For this review, use the dimensioned drawing (mm, ordinates from the lowest corner) and the shaded views. A direction names the side the tool comes from. Coordinates: 2 decimals unless noted, no trailing zeros. Loops run counter-clockwise (first coordinate to the right, second up) from the corner with the lowest first, then second, coordinate; pieces in that order, holes last. Notation, with made-up numbers: (88.5, 77) - (129.5, 77) arc R20 ccw to (129.5, 106) - close; hole circle Ø5 at (28.25, -16.75). An arc over 180 degrees is marked (long way). Use a Markdown table: item, result. Add a question column.
1) To check wall thickness, follow L1, parallel to Y at x = 19.05, z = 35.5; L2, parallel to X at y = 19, z = 30; L3, parallel to Z at x = 30.5, y = 83.5. State the ranges of each line that lie inside material, in increasing order. Write a range as [from, to].
2) Add section A-A, the plane z = 7.5. Give the boundary of the cut face in (x, y), and give its area (3 significant figures).
3) The part is to be moulded in two halves that separate along Y. For the marked faces 1, 2, 3 and 4, say which applies: pulls with the +Y half, pulls with the -Y half, needs draft (parallel to the pull), parting line crosses it, or undercut.
4) Add section C-C, the plane x = 19.05. Give the boundary of the cut face in (y, z) (3 decimals).
5) Clearance check with flat-ended pins moving along their axes: pin 1 (11.5 mm diameter, centred on x = 133.35, y = 19.05, fed in from -Z); pin 2 (14.5 mm diameter, centred on x = 91, y = 90.5, fed in from +Z); pin 3 (10 mm diameter, centred on x = 63, y = 74.5, fed in from -Z). State where each tip first meets the part, or that it passes through.
6) Add section B-B, the plane y = 19.05. Give the boundary of the cut face in (x, z).
7) For the marked faces 5, 6 and 7, list the 3-axis set-ups (+Z, -Z, +X, -X, +Y, -Y) from which the entire face can be reached by the end or side of a thin tool; tool diameter is ignored.
8) Add section D-D, the plane y = 42.5. Give the boundary of the cut face in (x, z), and give its area (3 significant figures).
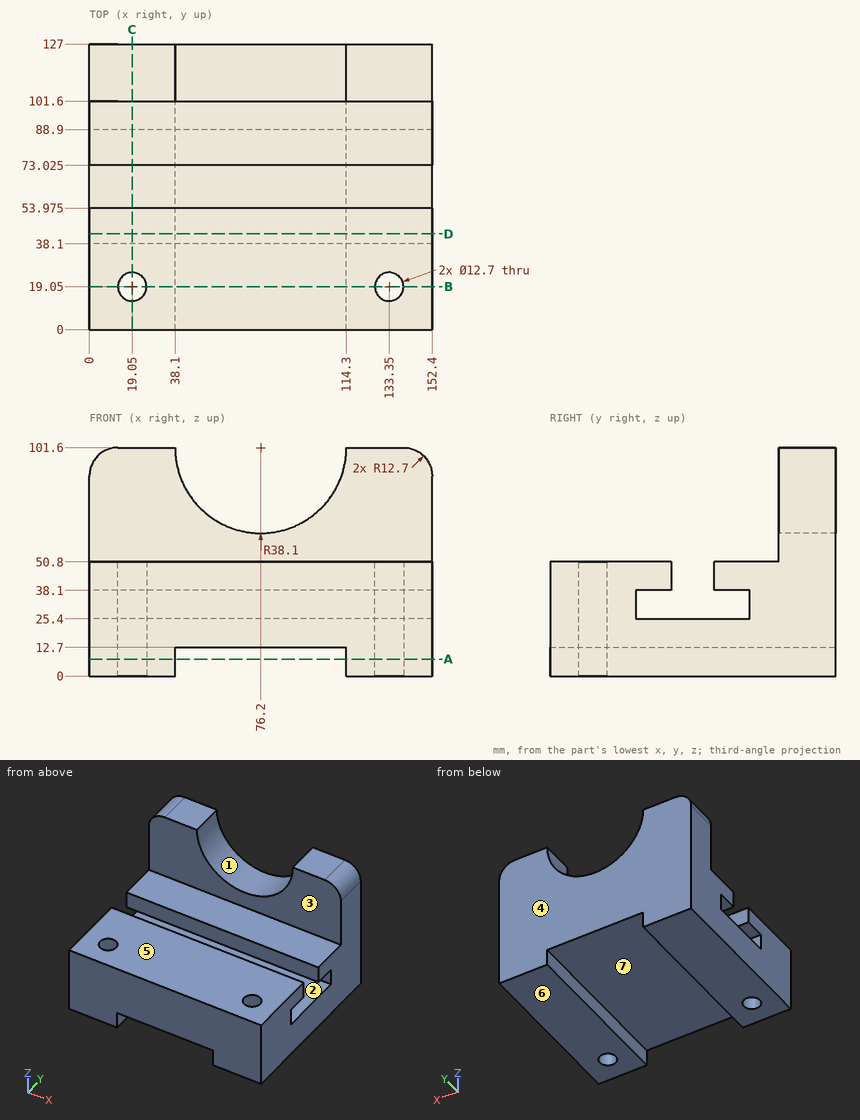
From the geometry:
| question | item | result |
|---|---|---|
| 1 | L1 | y = [0, 12.7], [25.4, 38.1], [88.9, 127] |
| 1 | L2 | x = [0, 12.7], [25.4, 127], [139.7, 152.4] |
| 1 | L3 | z = [0, 25.4], [38.1, 50.8] |
| 2 | outline | (0, 0) - (38.1, 0) - (38.1, 127) - (0, 127) - close; (114.3, 0) - (152.4, 0) - (152.4, 127) - (114.3, 127) - close; hole circle Ø12.7 at (19.05, 19.05); hole circle Ø12.7 at (133.35, 19.05) |
| 2 | area | 9,420 mm^2 |
| 3 | face 1 | needs draft |
| 3 | face 2 | undercut |
| 3 | face 3 | pulls with the -Y half |
| 3 | face 4 | pulls with the +Y half |
| 4 | outline | (0, 0) - (12.7, 0) - (12.7, 50.8) - (0, 50.8) - close; (25.4, 0) - (127, 0) - (127, 101.6) - (101.6, 101.6) - (101.6, 50.8) - (73.025, 50.8) - (73.025, 38.1) - (88.9, 38.1) - (88.9, 25.4) - (38.1, 25.4) - (38.1, 38.1) - (53.975, 38.1) - (53.975, 50.8) - (25.4, 50.8) - close |
| 5 | pin 1 | passes through |
| 5 | pin 2 | stops at z = 50.8 |
| 5 | pin 3 | stops at z = 12.7 |
| 6 | outline | (0, 0) - (12.7, 0) - (12.7, 50.8) - (0, 50.8) - close; (25.4, 0) - (38.1, 0) - (38.1, 12.7) - (114.3, 12.7) - (114.3, 0) - (127, 0) - (127, 50.8) - (25.4, 50.8) - close; (139.7, 0) - (152.4, 0) - (152.4, 50.8) - (139.7, 50.8) - close |
| 7 | face 5 | +Z, +X, -X, -Y |
| 7 | face 6 | -Z, +X, -X, +Y, -Y |
| 7 | face 7 | -Z, +Y, -Y |
| 8 | outline | (0, 0) - (38.1, 0) - (38.1, 12.7) - (114.3, 12.7) - (114.3, 0) - (152.4, 0) - (152.4, 25.4) - (0, 25.4) - close; (0, 38.1) - (152.4, 38.1) - (152.4, 50.8) - (0, 50.8) - close |
| 8 | area | 4,840 mm^2 |
